Read the model definition and answer for the solid it produces. Units are mm, in the model's axes. Face numbers are marked on the shaded views. A direction names the side the tool comes from. Coordinates: 2 decimals unless noted, no trailing zeros. Loops run counter-clockwise (first coordinate to the right, second up) from the corner with the lowest first, then second, coordinate; pieces in that order, holes last. Notation, with made-up numbers: M 60,4 L 113,4 A32 cw 113,34 Z; hole C 2,59.25 d8. An arc over 180 degrees is marked long. Use one line per item in the form item = value. Start each with the question number.
1. Flat-ended cylindrical pins translate along their axes: pin 1 (1.5 mm diameter, centred on y = 10, z = 4.5, fed in from +X); pin 2 (3 mm diameter, centred on x = -62, y = 0, fed in from -Z); pin 3 (2 mm diameter, centred on x = -52, y = -1, fed in from -Z); pin 4 (0.8 mm diameter, centred on x = -109, y = -12.5, fed in from -Z). Find the tip coordinate at first contact, or state that the pin passes through.
2. The part is cut by section C-C (x = -93). Give the vertices of the cut face in (y, z), plus the area to 3 significant figures.
3. A tool of negligible diameter and unlimited length cuts with its end or side. For the marked faces 4 and 5, from which of +Z, -Z, +X, -X, +Y, -Y can it reach the whole face along a straight path? Write none if from no direction.
4. The part is cut by section A-A (z = 2.25). Give the number of separate pieces and of enclosed holes in the cut face, plus the area to 3 significant figures.
5. For a pull along Y with two mould halves and no side action, classify the marked faces 1, 2 and 3 as released by +Y, released by -Y, zero draft, split by the parting line, or undercut.
6. Find the intervals of material crossed by probe 1 along X at (y, z) = (5.25, 1.35); probe 2 along Y at (x, z) = (-2.4, 2.25); probe 3 along Y at (x, z) = (-62, 3.7), in increasing order. Write a range as [from, to].
7. The part is cut by section D-D (x = -23.5). Give the vertices of the cut face in (y, z).
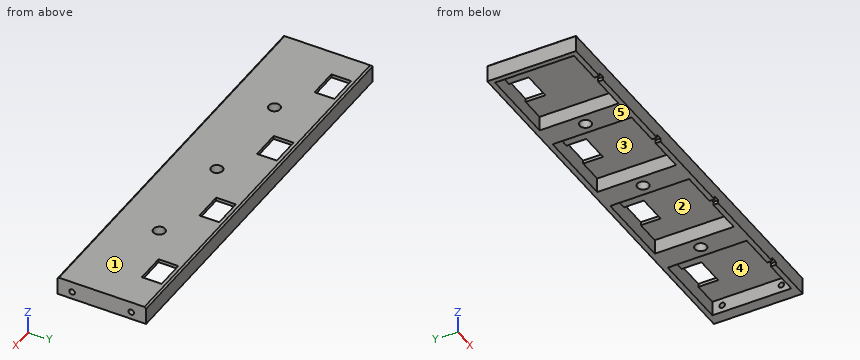
Autodesk Inventor part; units mm, degrees
ref_plane "YZ Plane" through (0, 0, 0) normal (1, 0, 0) x (0, 1, 0)
ref_plane "XZ Plane" through (0, 0, 0) normal (0, 1, 0) x (-1, 0, 0)
ref_plane "XY Plane" through (0, 0, 0) normal (0, 0, 1) x (1, 0, 0)
sketch "Sketch1" plane through (0, 0, 0) normal (0, 0, 1) x (1, 0, 0)
  line L0 (-122, 13.5) -> (122, 13.5)
  line L1 (122, 13.5) -> (122, -13.5)
  line L2 (122, -13.5) -> (-122, -13.5)
  line L3 (-122, -13.5) -> (-122, 13.5)
  line L4 (-122, 13.5) -> (122, -13.5) construction
  line L5 (122, 13.5) -> (-122, -13.5) construction
  line L6 (-120.5, -12) -> (-96.5, -12)
  line L7 (-96.5, -12) -> (-96.5, 12)
  line L8 (-96.5, 12) -> (-120.5, 12)
  line L9 (-120.5, 12) -> (-120.5, -12)
  line L10 (-120.5, -12) -> (-96.5, 12) construction
  line L11 (-96.5, -12) -> (-120.5, 12) construction
  line L12 (-122, 0) -> (-108.5, 0) construction
  line L13 (-89.5, -12) -> (-65.5, -12)
  line L14 (-65.5, -12) -> (-65.5, 12)
  line L15 (-65.5, 12) -> (-89.5, 12)
  line L16 (-89.5, 12) -> (-89.5, -12)
  line L17 (-89.5, -12) -> (-65.5, 12) construction
  line L18 (-65.5, -12) -> (-89.5, 12) construction
  line L19 (-58.5, -12) -> (-34.5, -12)
  line L20 (-34.5, -12) -> (-34.5, 12)
  line L21 (-34.5, 12) -> (-58.5, 12)
  line L22 (-58.5, 12) -> (-58.5, -12)
  line L23 (-58.5, -12) -> (-34.5, 12) construction
  line L24 (-34.5, -12) -> (-58.5, 12) construction
  line L25 (-27.5, -12) -> (-3.5, -12)
  line L26 (-3.5, -12) -> (-3.5, 12)
  line L27 (-3.5, 12) -> (-27.5, 12)
  line L28 (-27.5, 12) -> (-27.5, -12)
  line L29 (-27.5, -12) -> (-3.5, 12) construction
  line L30 (-3.5, -12) -> (-27.5, 12) construction
  line L31 (3.5, -12) -> (27.5, -12)
  line L32 (27.5, -12) -> (27.5, 12)
  line L33 (27.5, 12) -> (3.5, 12)
  line L34 (3.5, 12) -> (3.5, -12)
  line L35 (3.5, -12) -> (27.5, 12) construction
  line L36 (27.5, -12) -> (3.5, 12) construction
  line L37 (34.5, -12) -> (58.5, -12)
  line L38 (58.5, -12) -> (58.5, 12)
  line L39 (58.5, 12) -> (34.5, 12)
  line L40 (34.5, 12) -> (34.5, -12)
  line L41 (34.5, -12) -> (58.5, 12) construction
  line L42 (58.5, -12) -> (34.5, 12) construction
  line L43 (65.5, -12) -> (89.5, -12)
  line L44 (89.5, -12) -> (89.5, 12)
  line L45 (89.5, 12) -> (65.5, 12)
  line L46 (65.5, 12) -> (65.5, -12)
  line L47 (65.5, -12) -> (89.5, 12) construction
  line L48 (89.5, -12) -> (65.5, 12) construction
  line L49 (96.5, -12) -> (120.5, -12)
  line L50 (120.5, -12) -> (120.5, 12)
  line L51 (120.5, 12) -> (96.5, 12)
  line L52 (96.5, 12) -> (96.5, -12)
  line L53 (96.5, -12) -> (120.5, 12) construction
  line L54 (120.5, -12) -> (96.5, 12) construction
  point P0 (0, 0)
  point P1 (-77.5, 0)
  point P2 (-46.5, 0)
  point P3 (-15.5, 0)
  point P4 (15.5, 0)
  point P5 (46.5, 0)
  point P6 (77.5, 0)
  point P7 (108.5, 0)
  dimension "d2" = 24
  dimension "d3" = 24
  dimension "d6" = 31
  dimension "d11" = 7
  dimension "d12" = 1.5
  dimension "d13" = 1.5
  dimension "d14" = 1.5
extrude "Extrusion1" add sketch "Sketch1" along normal blind 4.5
sketch "Sketch2" plane through (0, 0, 4.5) normal (0, 0, 1) x (1, 0, 0)
  line L0 (-120.5, 12) -> (-96.5, 12) construction
  line L1 (-113, 6) -> (-104, 6)
  line L2 (-104, 6) -> (-104, 12)
  line L3 (-104, 12) -> (-113, 12)
  line L4 (-113, 12) -> (-113, 6)
  line L5 (-113, 6) -> (-104, 12) construction
  line L6 (-104, 6) -> (-113, 12) construction
  line L7 (-108.5, 12) -> (-108.5, 9) construction
  line L8 (122, 13.5) -> (-122, 13.5)
  line L9 (-122, -13.5) -> (122, -13.5)
  line L10 (-122, 13.5) -> (122, 13.5)
  line L11 (122, 13.5) -> (122, -13.5)
  line L12 (122, -13.5) -> (-122, -13.5)
  line L13 (-122, -13.5) -> (-122, 13.5)
  line L14 (-82, 6) -> (-73, 6)
  line L15 (-73, 6) -> (-73, 12)
  line L16 (-73, 12) -> (-82, 12)
  line L17 (-82, 12) -> (-82, 6)
  line L18 (-82, 6) -> (-73, 12) construction
  line L19 (-73, 6) -> (-82, 12) construction
  line L20 (-77.5, 12) -> (-77.5, 9) construction
  line L21 (-51, 6) -> (-42, 6)
  line L22 (-42, 6) -> (-42, 12)
  line L23 (-42, 12) -> (-51, 12)
  line L24 (-51, 12) -> (-51, 6)
  line L25 (-51, 6) -> (-42, 12) construction
  line L26 (-42, 6) -> (-51, 12) construction
  line L27 (-46.5, 12) -> (-46.5, 9) construction
  line L28 (-20, 6) -> (-11, 6)
  line L29 (-11, 6) -> (-11, 12)
  line L30 (-11, 12) -> (-20, 12)
  line L31 (-20, 12) -> (-20, 6)
  line L32 (-20, 6) -> (-11, 12) construction
  line L33 (-11, 6) -> (-20, 12) construction
  line L34 (-15.5, 12) -> (-15.5, 9) construction
  line L35 (11, 6) -> (20, 6)
  line L36 (20, 6) -> (20, 12)
  line L37 (20, 12) -> (11, 12)
  line L38 (11, 12) -> (11, 6)
  line L39 (11, 6) -> (20, 12) construction
  line L40 (20, 6) -> (11, 12) construction
  line L41 (15.5, 12) -> (15.5, 9) construction
  line L42 (42, 6) -> (51, 6)
  line L43 (51, 6) -> (51, 12)
  line L44 (51, 12) -> (42, 12)
  line L45 (42, 12) -> (42, 6)
  line L46 (42, 6) -> (51, 12) construction
  line L47 (51, 6) -> (42, 12) construction
  line L48 (46.5, 12) -> (46.5, 9) construction
  line L49 (73, 6) -> (82, 6)
  line L50 (82, 6) -> (82, 12)
  line L51 (82, 12) -> (73, 12)
  line L52 (73, 12) -> (73, 6)
  line L53 (73, 6) -> (82, 12) construction
  line L54 (82, 6) -> (73, 12) construction
  line L55 (77.5, 12) -> (77.5, 9) construction
  line L56 (104, 6) -> (113, 6)
  line L57 (113, 6) -> (113, 12)
  line L58 (113, 12) -> (104, 12)
  line L59 (104, 12) -> (104, 6)
  line L60 (104, 6) -> (113, 12) construction
  line L61 (113, 6) -> (104, 12) construction
  line L62 (108.5, 12) -> (108.5, 9) construction
  line L63 (-89.5, 12) -> (-65.5, 12) construction
  line L64 (-89.5, 12) -> (-65.5, 12) construction
  point P0 (0, 0)
  dimension "d17" = 6
  dimension "d18" = 9
  dimension "d21" = 31
extrude "Extrusion2" add sketch "Sketch2" along normal blind 1
sketch "Sketch3" plane through (0, 0, 0) normal (0, 0, -1) x (-1, 0, 0)
  line L0 (-96.5, -12) -> (-96.5, 12)
  line L1 (-96.5, 0) -> (-89.5, 0) construction
  line L2 (-89.5, 12) -> (-89.5, -12)
  circle A0 centre (-93, 0) radius 1.75
  line L3 (-65.5, -12) -> (-65.5, 12)
  line L4 (-65.5, 0) -> (-58.5, 0) construction
  line L5 (-58.5, 12) -> (-58.5, -12)
  circle A1 centre (-62, 0) radius 1.75
  circle A2 centre (-31, 0) radius 1.75
  circle A3 centre (0, 0) radius 1.75
  circle A4 centre (31, 0) radius 1.75
  circle A5 centre (62, 0) radius 1.75
  circle A6 centre (93, 0) radius 1.75
  point P0 (0, 0)
  dimension "d28" = 3.5
  dimension "d31" = 31
extrude "Extrusion3" cut sketch "Sketch3" against normal through all contours A0 | A1 | A2 | A4 | A5 | A6
sketch "Sketch4" plane through (-122, -13.5, 0) normal (0, -1, 0) x (1, 0, 0)
  line L0 (242.5, 0) -> (218.5, 0)
  line L1 (211.5, 0) -> (187.5, 0)
  line L2 (231.5, 1) -> (229.5, 1)
  line L3 (229.5, 1) -> (229.5, -1)
  line L4 (229.5, -1) -> (231.5, -1)
  line L5 (231.5, -1) -> (231.5, 1)
  line L6 (231.5, 1) -> (229.5, -1) construction
  line L7 (229.5, 1) -> (231.5, -1) construction
  line L8 (200.5, 1) -> (198.5, 1)
  line L9 (198.5, 1) -> (198.5, -1)
  line L10 (198.5, -1) -> (200.5, -1)
  line L11 (200.5, -1) -> (200.5, 1)
  line L12 (200.5, 1) -> (198.5, -1) construction
  line L13 (198.5, 1) -> (200.5, -1) construction
  line L14 (169.5, 1) -> (167.5, 1)
  line L15 (167.5, 1) -> (167.5, -1)
  line L16 (167.5, -1) -> (169.5, -1)
  line L17 (169.5, -1) -> (169.5, 1)
  line L18 (169.5, 1) -> (167.5, -1) construction
  line L19 (167.5, 1) -> (169.5, -1) construction
  line L20 (138.5, 1) -> (136.5, 1)
  line L21 (136.5, 1) -> (136.5, -1)
  line L22 (136.5, -1) -> (138.5, -1)
  line L23 (138.5, -1) -> (138.5, 1)
  line L24 (138.5, 1) -> (136.5, -1) construction
  line L25 (136.5, 1) -> (138.5, -1) construction
  line L26 (107.5, 1) -> (105.5, 1)
  line L27 (105.5, 1) -> (105.5, -1)
  line L28 (105.5, -1) -> (107.5, -1)
  line L29 (107.5, -1) -> (107.5, 1)
  line L30 (107.5, 1) -> (105.5, -1) construction
  line L31 (105.5, 1) -> (107.5, -1) construction
  line L32 (76.5, 1) -> (74.5, 1)
  line L33 (74.5, 1) -> (74.5, -1)
  line L34 (74.5, -1) -> (76.5, -1)
  line L35 (76.5, -1) -> (76.5, 1)
  line L36 (76.5, 1) -> (74.5, -1) construction
  line L37 (74.5, 1) -> (76.5, -1) construction
  line L38 (45.5, 1) -> (43.5, 1)
  line L39 (43.5, 1) -> (43.5, -1)
  line L40 (43.5, -1) -> (45.5, -1)
  line L41 (45.5, -1) -> (45.5, 1)
  line L42 (45.5, 1) -> (43.5, -1) construction
  line L43 (43.5, 1) -> (45.5, -1) construction
  line L44 (14.5, 1) -> (12.5, 1)
  line L45 (12.5, 1) -> (12.5, -1)
  line L46 (12.5, -1) -> (14.5, -1)
  line L47 (14.5, -1) -> (14.5, 1)
  line L48 (14.5, 1) -> (12.5, -1) construction
  line L49 (12.5, 1) -> (14.5, -1) construction
  point P0 (122, 0)
  point P1 (230.5, 0)
  point P2 (199.5, 0)
  point P3 (168.5, 0)
  point P4 (137.5, 0)
  point P5 (106.5, 0)
  point P6 (75.5, 0)
  point P7 (44.5, 0)
  point P8 (13.5, 0)
  dimension "d40" = 31
  dimension "d45" = 1
  dimension "d46" = 2
extrude "Extrusion4" cut sketch "Sketch4" against normal blind 4.5
sketch "Sketch5" plane through (-3.5, -12, 0) normal (-1, 0, 0) x (0, 0, 1)
  line L0 (0, 0) -> (4.5, 0)
  line L1 (2.25, 0) -> (2.25, 24) construction
  line L2 (0, 24) -> (4.5, 24)
  circle A0 centre (2.25, 3) radius 0.85
  circle A1 centre (2.25, 21) radius 0.85
  point P0 (0, 12)
  dimension "d49" = 1.7
  dimension "d50" = 3
  dimension "d51" = 3
extrude "Extrusion5" cut sketch "Sketch5" against normal up to surface (7 mm away)
chamfer "Chamfer1" distance 0.5 angle 45 4 edges at (0, -13.5, 5.5) (122, 0, 5.5) (0, 13.5, 5.5) (-122, 0, 5.5)
sketch "Sketch7" plane through (0, 0, 0) normal (0, 0, -1) x (-1, 0, 0)
  line L0 (-167.9022, 73.2731) -> (0, 73.2731)
  line L1 (0, 73.2731) -> (0, -62.2269)
  line L2 (0, -62.2269) -> (-167.9022, -62.2269)
  line L3 (-167.9022, -62.2269) -> (-167.9022, 73.2731)
  line L4 (0, 73.2731) -> (150.1362, 73.2731)
  line L5 (150.1362, 73.2731) -> (150.1362, -62.2269)
  line L6 (150.1362, -62.2269) -> (0, -62.2269)
  line L7 (0, -62.2269) -> (0, 73.2731)
  point P0 (0, 0)
extrude "Extrusion7" cut sketch "Sketch7" against normal through all contours L0 L1 L2 L3
properties part number "SensorHolder"
Computed values:
q1.pin_1 = 0
q1.pin_2 = through
q1.pin_3 = 4.5
q1.pin_4 = 1
q2.outline = M -13.5,0 L -1.75,0 L -1.75,5.5 L -13,5.5 L -13.5,5 Z; M 1.75,0 L 13.5,0 L 13.5,5 L 13,5.5 L 1.75,5.5 Z
q2.area = 129 mm²
q3.face_4 = -Z
q3.face_5 = -Z, +X, -X, +Y, -Y
q4.separate_pieces = 2
q4.enclosed_holes = 6
q4.area = 949 mm²
q5.face_1 = zero draft
q5.face_2 = undercut
q5.face_3 = undercut
q6.probe_1 = [-122, -120.5], [-96.5, -89.5], [-65.5, -58.5], [-34.5, -27.5], [-3.5, 0]
q6.probe_2 = [-13.5, -9.85], [-8.15, 8.15], [9.85, 13.5]
q6.probe_3 = [-13.5, -1.75], [1.75, 13.5]
q7.outline = M -13.5,0 L -12,0 L -12,4.5 L 12,4.5 L 12,0 L 13.5,0 L 13.5,5 L 13,5.5 L -13,5.5 L -13.5,5 Z
